Source: three-view drawing plus pictorial views. Frame: mm from the lowest corner of the part. A direction names the side the tool comes from. Give positions to 0.01 mm unless a question says otherwise; leave off trailing zeros. Write each loop counter-clockwise with the first axis right and the second up, starting at its lowest first coordinate (ties: lowest second). Pieces come first, ordered by that corner, then holes.
Q1. Line query: L1, parallel to X at y = 66.5, z = 346; L2, parallel to Y at x = 261, z = 450; L3, parallel to X at y = 76, z = 295. Output: solid intervals per line, ascending.
Q2. Reachability of the marked faces 1 and 2 from +Z, -Z, +X, -X, +Y, -Y: full face, straight path, thin tool, end or side. Return the list, or none.
Q3. Draft query along X for the marked faces 3, 4, 5 and 6. Return one class per face: pulls with the +X half, pulls with the -X half, needs draft (parallel to the pull), parting line crosses it, or undercut.
Q4. Cut plane A-A on z = 450. Return the cut outline in (x, y).
Q5. Cut plane C-C on x = 150. Return the cut outline in (y, z).
Q6. Cut plane D-D on z = 358. Return the cut outline in (x, y).
Q7. Cut plane B-B on y = 75. Return the cut outline in (x, z), plus the area to 3 significant figures.
Q8. Pin query (flat end, axial travel): pin 1 (5 mm diameter, centred on x = 99.5, y = 63.5, fed in from -Z); pin 2 (2 mm diameter, centred on x = 137, y = 79, fed in from +Z); pin 3 (4 mm diameter, centred on x = 161.5, y = 64, fed in from -Z). Return the tip coordinate at first contact, or that it passes through.
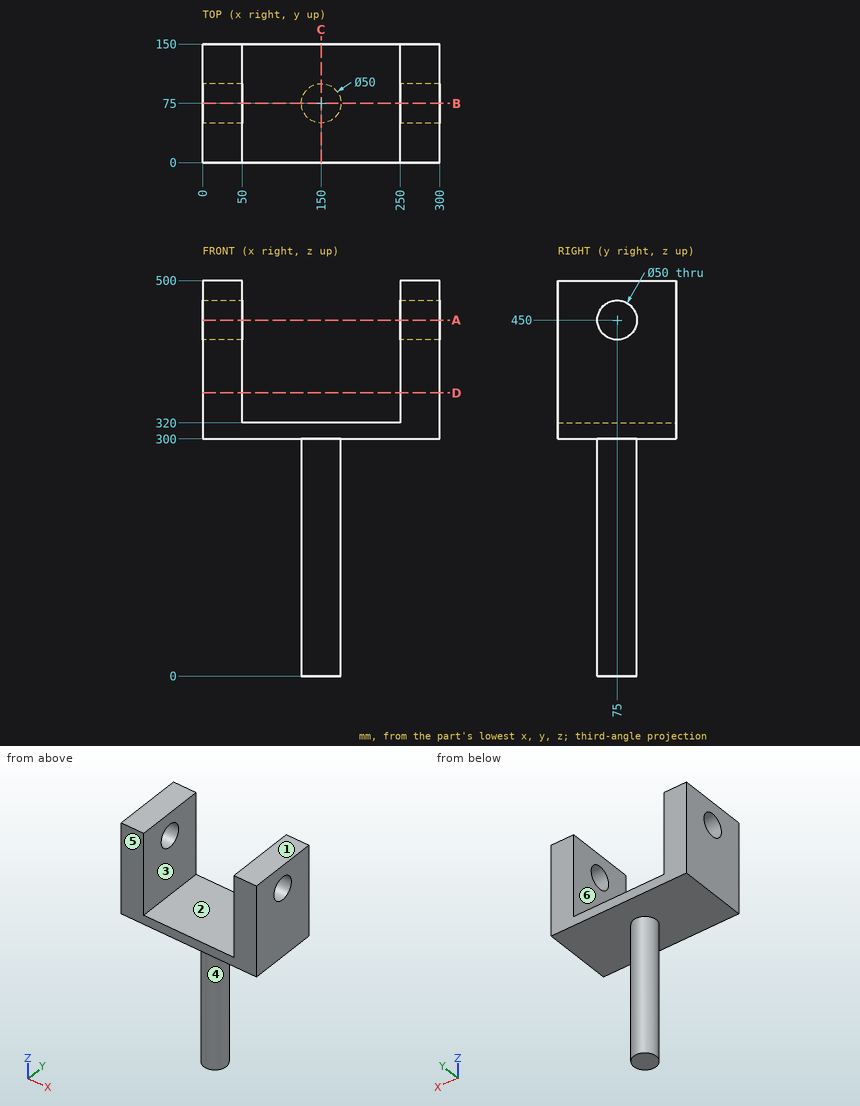
Data:
1. L1: x = 0 to 50, 250 to 300
1. L2: y = 0 to 50, 100 to 150
1. L3: x = 125.02 to 174.98
2. face 1: +Z, +X, -X, +Y, -Y
2. face 2: +Z, +Y, -Y
3. face 3: undercut
3. face 4: parting line crosses it
3. face 5: needs draft
3. face 6: undercut
4. outline: (0, 0) - (50, 0) - (50, 50) - (0, 50) - close; (0, 100) - (50, 100) - (50, 150) - (0, 150) - close; (250, 0) - (300, 0) - (300, 50) - (250, 50) - close; (250, 100) - (300, 100) - (300, 150) - (250, 150) - close
5. outline: (0, 300) - (50, 300) - (50, 0) - (100, 0) - (100, 300) - (150, 300) - (150, 320) - (0, 320) - close
6. outline: (0, 0) - (50, 0) - (50, 150) - (0, 150) - close; (250, 0) - (300, 0) - (300, 150) - (250, 150) - close
7. outline: (0, 300) - (125, 300) - (125, 0) - (175, 0) - (175, 300) - (300, 300) - (300, 425) - (250, 425) - (250, 320) - (50, 320) - (50, 425) - (0, 425) - close; (0, 475) - (50, 475) - (50, 500) - (0, 500) - close; (250, 475) - (300, 475) - (300, 500) - (250, 500) - close
7. area: 34,000 mm2
8. pin 1: stops at z = 300
8. pin 2: stops at z = 320
8. pin 3: stops at z = 0
